```python
from build123d import *

# Parameters (mm, degrees)
SKETCH_1_R          = 1.5
SKETCH_1_W          = 8
SKETCH_1_H          = 6
EXTRUDE_2_DEPTH     = 6
SKETCH_1_4_W        = 8
SKETCH_1_4_H        = 3
EXTRUDE_3_DEPTH     = 3
EXTRUDE_28_DEPTH    = 8
SKETCH_4_W          = 7.960549586
SKETCH_4_H          = 11.5
EXTRUDE_29_DEPTH    = 18
EXTRUDE_30_DEPTH    = 36
SKETCH_8_R          = 1.9
CUT_EXTRUDE_2_DEPTH = 19
SKETCH_7_R          = 1.5
CUT_EXTRUDE_3_DEPTH = 10


with BuildPart() as part:
    # Sketch 1 → Extrude 2 (new body)
    # profile 1 of 2: a face of its own
    with BuildSketch(Plane(origin=(0, 0, 0), x_dir=(1, 0, 0), z_dir=(0, 1, 0))):
        with BuildLine():
            Line((-38.676968887, 3), (-6.676968887, 3))
            ThreePointArc((-6.676968887, 3), (-3.676968887, 0), (-6.676968887, -3))
            Line((-6.676968887, -3), (-38.676968887, -3))
            ThreePointArc((-38.676968887, -3), (-41.676968887, 0), (-38.676968887, 3))
        make_face()
        with Locations(Location((-6.676968887, 0, 0), (0, 0, 270))):
            Circle(SKETCH_1_R, mode=Mode.SUBTRACT)
        with Locations(Location((-38.676968887, 0, 0), (0, 0, 270))):
            Circle(SKETCH_1_R, mode=Mode.SUBTRACT)
    # profile 2 of 2: a face of its own
    with BuildSketch(Plane(origin=(0, 0, 0), x_dir=(1, 0, 0), z_dir=(0, 1, 0))):
        with Locations((-13.722758256, 0)):
            Rectangle(SKETCH_1_W, SKETCH_1_H)
    extrude(amount=-EXTRUDE_2_DEPTH)

    # Sketch 1_4 → Extrude 3 (add)
    with BuildSketch(Plane(origin=(0, 0, 0), x_dir=(1, 0, 0), z_dir=(0, 1, 0))):
        with Locations((-13.722758256, -1.5)):
            Rectangle(SKETCH_1_4_W, SKETCH_1_4_H)
        with Locations((-13.722758256, 1.5)):
            Rectangle(SKETCH_1_4_W, SKETCH_1_4_H)
    extrude(amount=EXTRUDE_3_DEPTH)

    # Sketch 3 → Extrude 28 (add)
    with BuildSketch(Plane(origin=(-9.722758256, 0, 0), x_dir=(0, 0, -1), z_dir=(1, 0, 0))):
        with BuildLine():
            Line((3, -2.291502622), (16.228756555, 12.708497378))
            ThreePointArc((16.228756555, 12.708497378), (15.874507866, 18.354248689), (10.228756555, 18))
            Line((10.228756555, 18), (-3, 3))
            Line((-3, 3), (3, -2.291502622))
        make_face()
    extrude(amount=-EXTRUDE_28_DEPTH)

    # Sketch 4 → Extrude 29 (add)
    with BuildSketch(Plane(origin=(0, -2.49076751, -2.824264888), x_dir=(-1, 0, 0), z_dir=(0, -0.6614378277661491, -0.7499999999999987))):
        with Locations((13.703033049, 8.211179299)):
            Rectangle(SKETCH_4_W, SKETCH_4_H)
    extrude(amount=EXTRUDE_29_DEPTH)

    # Sketch 6 → Extrude 30 (add)
    with BuildSketch(Plane.ZY.offset(17.683307842)):
        Polygon((-25.558716996, -3.925763935), (-17.952181977, -12.550763935), (-13.452181977, -8.582136969), (-21.058716996, 0.042863031), align=None)
    extrude(amount=-EXTRUDE_30_DEPTH)

    # Sketch 8 → Cut-Extrude 2 (cut)
    with BuildSketch(Plane(origin=(-9.722758256, 0, 0), x_dir=(0, 0, -1), z_dir=(1, 0, 0))):
        with Locations((13.228756555, 15.354248689)):
            Circle(SKETCH_8_R)
    extrude(amount=-CUT_EXTRUDE_2_DEPTH, mode=Mode.SUBTRACT)

    # Sketch 7 → Cut-Extrude 3 (cut)
    with BuildSketch(Plane(origin=(0, -14.396648409, -16.324264888), x_dir=(-1, 0, 0), z_dir=(0, -0.6614378277661491, -0.7499999999999987))):
        with Locations(Location((2.344835531, 8.278010001, 0), (0, 0, 90))):
            Circle(SKETCH_7_R)
        with Locations(Location((-15.655164469, 8.278010001, 0), (0, 0, 90))):
            Circle(SKETCH_7_R)
    extrude(amount=-CUT_EXTRUDE_3_DEPTH, mode=Mode.SUBTRACT)


solid = part.part
```
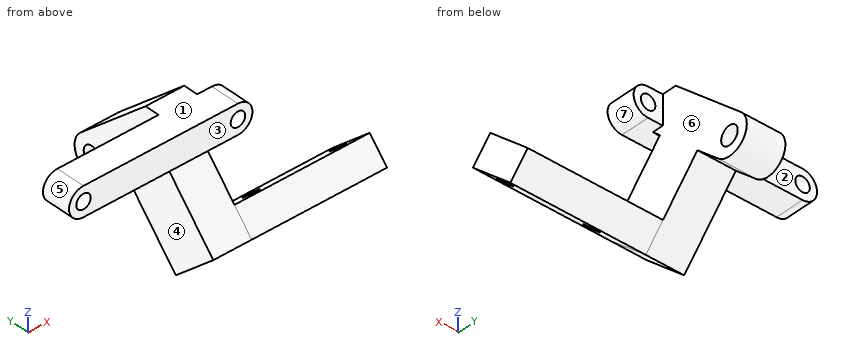
Could you check a few things on this model? Use its own coordinates, in mm. Face numbers are marked on the shaded views. A direction names the side the tool comes from. Round coordinates to 2 decimals unless told otherwise and drop trailing zeros. Loops run counter-clockwise (first coordinate to the right, second up) from the corner with the lowest first, then second, coordinate; pieces in that order, holes last. Notation, with made-up numbers: (73.25, 41.5) -> (95.25, 41.5) arc R30 cw to (95.25, 70.5) -> close; hole circle Ø8 at (60, 25.25). An arc over 180 degrees is marked (long way). Put each result on its own line as item: value.
Q1. I want a section at B-B on x = -27.5. Write out the boundary of the cut face in (y, z).
Checks:
outline: (-6, -3) -> (0, -3) -> (0, 3) -> (-6, 3) -> close
Q2. I want a section at A-A on z = 0.5. Write out the boundary of the cut face in (x, y) (3 decimals).
Checks:
outline: (-41.635, -6) -> (-40.091, -6) -> (-40.091, 0) -> (-41.635, 0) -> close; (-37.263, -6) -> (-8.091, -6) -> (-8.091, 0) -> (-9.723, 0) -> (-9.723, 5.835) -> (-17.723, 5.835) -> (-17.723, 0) -> (-37.263, 0) -> close; (-5.263, -6) -> (-3.719, -6) -> (-3.719, 0) -> (-5.263, 0) -> close
Q3. For pin 1 Ø6 at (y, z) = (12, -2.5) entering from -X; pin 2 Ø6 at (x, z) = (-14.5, -5) entering from +Y; pin 3 Ø5 at (x, z) = (-38.68, 0) entering from +Y; pin 4 Ø1.8 at (x, z) = (-6.68, 0) entering from +Y, each with a flat end and sliding along its axis, tell me the tip position at first contact or that it passes through.
Checks:
pin 1: x = -17.72
pin 2: y = 15.47
pin 3: y = 0
pin 4: through
Q4. Please list where these lines run through material, in increasing order: line 1 (X direction, y = -3.2, z = 0); line 2 (Y direction, x = -12, z = -14.75); line 3 (Y direction, x = -8.5, z = -1.5). Write a range as from..to.
Checks:
line 1: -41.68..-40.18, -37.18..-8.18, -5.18..-3.68
line 2: -9.73..5.61, 11.03..14.22, 16.49..19.05
line 3: -6..0
Q5. Which directions (+Z, -Z, +X, -X, +Y, -Y) give clear straight access to the entire face, cutting with the end or side of a thin tool? Please do the marked faces 1, 2 and 3.
Checks:
face 1: +Z, +X, -X, +Y, -Y
face 2: +Z, -Z, -X, +Y
face 3: +Z, +X, -X, -Y
Q6. Thinking about a two-plate mould opening in Z: for the marked faces 4, 5, 6 and 7, which applies, pulls with the +Z half, pulls with the -Z half, needs draft (parallel to the pull), parting line crosses it, or undercut?
Checks:
face 4: needs draft
face 5: parting line crosses it
face 6: undercut
face 7: undercut
